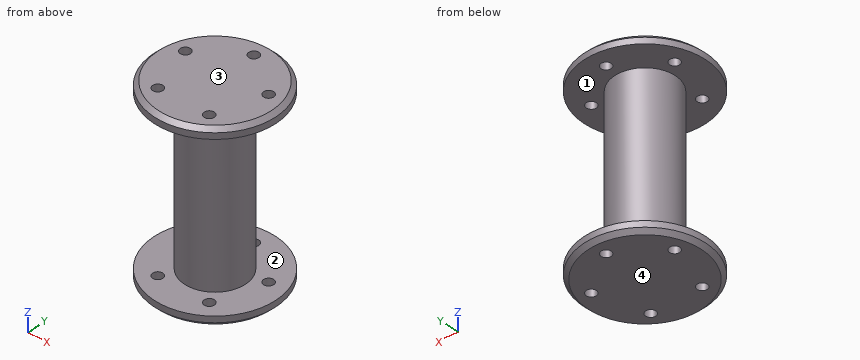
from build123d import *

# Parameters (mm, degrees)
SKETCH1_R             = 15
BOSS_EXTRUDE1_DEPTH   = 80
SKETCH2_R             = 30
BOSS_EXTRUDE2_DEPTH   = 5
CHAMFER1_SIZE         = 2
SKETCH3_R             = 2.5
CUT_EXTRUDE1_DEPTH    = 96
CIRPATTERN5_START     = -5
CIRPATTERN5_OUTLINE_R = 2.5
CIRPATTERN5_DEPTH     = 5


# Read off the part's stored shape, not the designer's step: CirPattern5, Mirror3
with BuildPart() as part:
    # Sketch1 → Boss-Extrude1 (new body)
    with BuildSketch(Plane.XY):
        Circle(SKETCH1_R)
    extrude(amount=BOSS_EXTRUDE1_DEPTH)

    # Sketch2 → Boss-Extrude2 (add)
    with BuildSketch(Plane(origin=(0, 0, 0), x_dir=(-1, 0, 0), z_dir=(0, 0, -1))):
        Circle(SKETCH2_R)
    extrude(amount=BOSS_EXTRUDE2_DEPTH)

    # Chamfer1
    chamfer1_edges = [part.edges().sort_by_distance(p)[0] for p in [
        (30, 0, -5),
    ]]
    chamfer(chamfer1_edges, length=CHAMFER1_SIZE)

    # Sketch3 → Cut-Extrude1 (cut, through all)
    with BuildSketch(Plane(origin=(0, 0, -5), x_dir=(-1, 0, 0), z_dir=(0, 0, -1))):
        with Locations((0, 21.5)):
            Circle(SKETCH3_R)
    extrude(amount=-CUT_EXTRUDE1_DEPTH, mode=Mode.SUBTRACT)

    # CirPattern5 outline → CirPattern5 (cut)
    with BuildSketch(Plane.XY.offset(CIRPATTERN5_START)):
        with Locations((20.4477151, 6.643865379)):
            Circle(CIRPATTERN5_OUTLINE_R)
        with Locations((12.637382924, -17.393865379)):
            Circle(CIRPATTERN5_OUTLINE_R)
        with Locations((-12.637382924, -17.393865379)):
            Circle(CIRPATTERN5_OUTLINE_R)
        with Locations((-20.4477151, 6.643865379)):
            Circle(CIRPATTERN5_OUTLINE_R)
    extrude(amount=CIRPATTERN5_DEPTH, mode=Mode.SUBTRACT)

    # Mirror3: part across plane


with BuildPart() as part_1:
    add(part.part)
    add(part.part.mirror(Plane.XY.offset(40)))


solid = part_1.part
Source: CAD feature listing. Evaluate the final solid. Frame: model axes, mm. Face numbers are marked on the shaded views. Give positions to 0.01 mm unless a question says otherwise; leave off trailing zeros. Order: outer loops, then holes, each group sorted by start corner. A loop starts at its lowest first (then second) coordinate and runs counter-clockwise, first axis right, second up. Notation, with made-up numbers: (69, 72) -> (106, 72) arc R23 cw to (106, 84) -> close; hole circle Ø8 at (-32, 36). An arc over 180 degrees is marked (long way). Write item = value, one per line.
Item 1: Contact query for flat-ended pins moving along their axis: pin 1 (12 mm diameter, centred on y = -6.5, z = 35, fed in from -X); pin 2 (1.5 mm diameter, centred on y = 1.5, z = 60.5, fed in from +X); pin 3 (10 mm diameter, centred on x = 8, z = 30.5, fed in from -Y). Output: stop coordinate, or through.
Check result:
pin_1 = -14.99
pin_2 = 14.98
pin_3 = -14.7
Item 2: Section query D-D (y = 21.5). State how many separate pieces and enclosed holes the cut face has, then the cut area to 3 significant figures.
Check result:
separate_pieces = 4
enclosed_holes = 0
area = 357 mm²
Item 3: Section query C-C (z = 32). Output: boundary loops of the cut face in (x, y), then the cut area to 3 significant figures.
Check result:
outline = circle Ø30 at (0, 0)
area = 707 mm²
Item 4: Ray query, probe 1 along Z at (x, y) = (20.5, -10); probe 2 along X at (y, z) = (-0.5, 4); probe 3 along Z at (x, y) = (-20, -21). Return the intervals inside material, ascending.
Check result:
probe_1 = -5 to 0, 80 to 85
probe_2 = -14.99 to 14.99
probe_3 = -4 to 0, 80 to 84
Item 5: Section query B-B (y = 0). Output: boundary loops of the cut face in (x, z).
Check result:
outline = (-30, -3) -> (-28, -5) -> (28, -5) -> (30, -3) -> (30, 0) -> (15, 0) -> (15, 80) -> (30, 80) -> (30, 83) -> (28, 85) -> (-28, 85) -> (-30, 83) -> (-30, 80) -> (-15, 80) -> (-15, 0) -> (-30, 0) -> close
Item 6: Section query A-A (x = 0). Output: boundary loops of the cut face in (y, z).
Check result:
outline = (-30, -3) -> (-28, -5) -> (19, -5) -> (19, 0) -> (15, 0) -> (15, 80) -> (19, 80) -> (19, 85) -> (-28, 85) -> (-30, 83) -> (-30, 80) -> (-15, 80) -> (-15, 0) -> (-30, 0) -> close; (24, -5) -> (28, -5) -> (30, -3) -> (30, 0) -> (24, 0) -> close; (24, 80) -> (30, 80) -> (30, 83) -> (28, 85) -> (24, 85) -> close
Item 7: Mould query, pull axis Z, two halves, no side actions, for the marked faces 1, 2, 3 and 4. Classes: +Z half, -Z half, draft (parallel to the pull), parting line (faces both ways), or undercut.
Check result:
face_1 = undercut
face_2 = undercut
face_3 = +Z half
face_4 = -Z half
